Check sheet for the modelled part. Datum: model origin and axes. Units: mm. A direction names the side the tool comes from. Round coordinates to 2 decimals unless told otherwise and drop trailing zeros. Write each loop counter-clockwise with the first axis right and the second up, starting at its lowest first coordinate (ties: lowest second). Pieces come first, ordered by that corner, then holes. Notation, with made-up numbers: M 39,89 L 45,89 A13 ccw 45,109 Z; hole C 63,57.5 d11. An arc over 180 degrees is marked long. One line per item, written item: value.
from build123d import *

# Parameters (mm, degrees)
SKETCH_1_R          = 1.5
SKETCH_1_W          = 10.2
SKETCH_1_H          = 10.2
EXTRUDE_1_DEPTH     = 2
SKETCH_2_R          = 0.5
CUT_EXTRUDE_1_DEPTH = 10
FILLET_1_R          = 1


with BuildPart() as part:
    # 草图1 → 凸台-拉伸1 (new body)
    with BuildSketch(Plane.XY):
        Polygon((5, 30), (-5, 30), (-5, -5), (40, -5), (40, 15), align=None)
        Circle(SKETCH_1_R, mode=Mode.SUBTRACT)
        with Locations((10.1, 10)):
            Rectangle(SKETCH_1_W, SKETCH_1_H, mode=Mode.SUBTRACT)
        with Locations((20, 0)):
            Circle(SKETCH_1_R, mode=Mode.SUBTRACT)
        with Locations((35, 0)):
            Circle(SKETCH_1_R, mode=Mode.SUBTRACT)
        with Locations((20, 10)):
            Circle(SKETCH_1_R, mode=Mode.SUBTRACT)
        with Locations((35, 10)):
            Circle(SKETCH_1_R, mode=Mode.SUBTRACT)
        with Locations((0, 25)):
            Circle(SKETCH_1_R, mode=Mode.SUBTRACT)
    extrude(amount=EXTRUDE_1_DEPTH)

    # 草图2 → 切除-拉伸1 (cut)
    with BuildSketch(Plane.XY.offset(2)):
        with Locations((15.2, 15.1)):
            Circle(SKETCH_2_R)
        with Locations((15.2, 4.9)):
            Circle(SKETCH_2_R)
        with Locations((5, 15.1)):
            Circle(SKETCH_2_R)
        with Locations((5, 4.9)):
            Circle(SKETCH_2_R)
    extrude(amount=-CUT_EXTRUDE_1_DEPTH, mode=Mode.SUBTRACT)

    # 圆角1
    fillet_1_edges = [part.edges().sort_by_distance(p)[0] for p in [
        (-5, 30, 1),
        (5, 30, 1),
        (40, 15, 1),
        (40, -5, 1),
        (-5, -5, 1),
    ]]
    fillet(fillet_1_edges, radius=FILLET_1_R)


solid = part.part
Q1. Sectioned sample at B-B on y = 0. Enter the section's corners in (x, z).
Completed:
outline: M -5,0 L -1.5,0 L -1.5,2 L -5,2 Z; M 1.5,0 L 18.5,0 L 18.5,2 L 1.5,2 Z; M 21.5,0 L 33.5,0 L 33.5,2 L 21.5,2 Z; M 36.5,0 L 40,0 L 40,2 L 36.5,2 Z
Q2. Sectioned sample at A-A on x = 0. Enter the section's corners in (y, z).
Completed:
outline: M -5,0 L -1.5,0 L -1.5,2 L -5,2 Z; M 1.5,0 L 23.5,0 L 23.5,2 L 1.5,2 Z; M 26.5,0 L 30,0 L 30,2 L 26.5,2 Z
Q3. Sectioned sample at D-D on y = 7. Enter the section's corners in (x, z).
Completed:
outline: M -5,0 L 5,0 L 5,2 L -5,2 Z; M 15.2,0 L 40,0 L 40,2 L 15.2,2 Z
Q4. Sectioned sample at C-C on z = 1.7. Enter the section's corners in (x, y).
Completed:
outline: M -5,-4 A1 ccw -4,-5 L 39,-5 A1 ccw 40,-4 L 40,14.34 A1 ccw 39.39,15.26 L 5.19,29.92 A1 ccw 4.79,30 L -4,30 A1 ccw -5,29 Z; hole C 0,0 d3; hole C 0,25 d3; hole M 5,5.4 A0.5 ccw long 5.5,4.9 L 14.7,4.9 A0.5 ccw long 15.2,5.4 L 15.2,14.6 A0.5 ccw long 14.7,15.1 L 5.5,15.1 A0.5 ccw long 5,14.6 Z; hole C 20,0 d3; hole C 20,10 d3; hole C 35,0 d3; hole C 35,10 d3
Q5. Scan lines: line 1 (X direction, y = 8, z = 1); line 2 (Y direction, x = 35, z = 0.5); line 3 (Y direction, x = 0.5, z = 1.3). Record each from-to range of solid material in increasing order. Write a range as [from, to].
Completed:
line 1: [-5, 5], [15.2, 40]
line 2: [-5, -1.5], [1.5, 8.5], [11.5, 17.14]
line 3: [-5, -1.41], [1.41, 23.59], [26.41, 30]
Q6. Access from +Z, -Z, +X, -X, +Y, -Y to the whole of each face (thin tool, end or side, straight path). Record for faces 1 (the flat face through (40, 5, 1)), 2 (the flat face through (5, 10, 1)).
Completed:
face 1: +Z, -Z, +X, +Y, -Y
face 2: +Z, -Z
Q7. Draft check along X on faces 3 (the cylindrical face through (18.5, 10.07, 0.99)), 4 (the flat face through (17, 9, 0)), 5 (the cylindrical face through (-4.699, 29.715, 1.014)), 6 (the cylindrical face through (18.5, 0.07, 0.99)). Enter one of: pulls with the +X half, pulls with the -X half, needs draft (parallel to the pull), parting line crosses it, or undercut.
Completed:
face 3: undercut
face 4: needs draft
face 5: pulls with the -X half
face 6: undercut
Q8. Depth check by flat-ended pin: P1, Ø1, axis at x = 10, z = 1, coming from the +Y side; P2, Ø3.5, axis at x = 35, y = 10, coming from the -Z side. Enter the tip coordinate at first touch or a pass-through.
Completed:
P1: y = 28.07
P2: z = 0
